Source: CAD feature listing. Evaluate the final solid. Frame: model axes, mm. A direction names the side the tool comes from. Round coordinates to 2 decimals unless told otherwise and drop trailing zeros. Order: outer loops, then holes, each group sorted by start corner. A loop starts at its lowest first (then second) coordinate and runs counter-clockwise, first axis right, second up. Notation, with made-up numbers: (-14.5, 63) - (37.5, 63) arc R11 ccw to (37.5, 81) - close; hole circle Ø11 at (49.25, 25.5). An arc over 180 degrees is marked (long way). Use one line per item in the form item = value. Start each with the question number.
Q1. Ray query, line 1 (X direction, y = 3.5, z = 0); line 2 (X direction, y = 4.75, z = 2.75); line 3 (Z direction, x = -0.25, y = 3.25). Return the intervals inside material, ascending. Write a range as [from, to].
Q2. Cut plane B-B, the plane x = 0. Return the cut outline in (y, z).
Q3. Pin query (flat end, axial travel): pin 1 Ø2 at (x, z) = (3.5, 5.5) entering from +Y; pin 2 Ø1 at (y, z) = (5.5, -5.5) entering from -X; pin 3 Ø6.5 at (x, z) = (0, 0) entering from +Y; pin 4 Ø1 at (x, y) = (5, 4.5) entering from -Z. Return the tip coordinate at first contact, or that it passes through.
Q4. Cut plane D-D, the plane x = -7. Return the cut outline in (y, z), and give its area (3 significant figures).
Q5. Set-up query: faces 5 (the flat face through (5.5, 3, 7)), 6 (the flat face through (6, 0, 0)). Return all of +Z, -Z, +X, -X, +Y, -Y with unobstructed straight access to the full face (end or side cutting, diameter ignored); none if empty.
Q6. Draft query along X for faces 1 (the cylindrical face through (-0.179, 2.958, -5.497)), 2 (the cylindrical face through (-7.02, 0.57, 7.9)), 3 (the cylindrical face through (-6.766, 2.958, -3.49)), 4 (the cylindrical face through (-0.1, 3, -7.5)). Return one class per face: released by +X, released by -X, zero draft, split by the parting line, or undercut.
Q7. Cut plane A-A, the plane z = 0. Return the cut outline in (x, y), and give its area (3 significant figures).
Q8. Cut plane C-C, the plane z = 2. Return the cut outline in (x, y), and give its area (3 significant figures).
Autodesk Inventor part; units mm, degrees
ref_plane "XZ Plane" through (0, 0, 0) normal (0, 1, 0) x (-1, 0, 0)
ref_plane "XY Plane" through (0, 0, 0) normal (0, 0, 1) x (1, 0, 0)
sketch "Sketch1" plane through (0, 0, 0) normal (0, 1, 0) x (-1, 0, 0)
  circle A0 centre (0, 0) radius 5.5
  circle A1 centre (0, 0) radius 7.5
  line L0 (7.5, 0) -> (-7.5, 0)
  line L1 (-7.5, 0) -> (-7.5, 8.5)
  line L2 (-7.5, 8.5) -> (7.5, 8.5)
  line L3 (7.5, 8.5) -> (7.5, 0)
  line L4 (5.5, 0) -> (-5.5, 0)
  line L5 (-5.5, 0) -> (-5.5, 8.5)
  line L6 (-5.5, 8.5) -> (5.5, 8.5)
  line L7 (5.5, 8.5) -> (5.5, 0)
  line L8 (4, 3.7749) -> (4, 6.3443)
  line L9 (-4, 3.7749) -> (-4, 6.3443)
  line L10 (4, 6.3443) -> (5.5, 6.3443)
  line L11 (-4, 6.3443) -> (-5.5, 6.3443)
  line L12 (-10.5, 0) -> (10.5, 0)
  point P0 (-5.5, 8.5)
  dimension "d0" = 11
  dimension "d1" = 2
  dimension "d3" = 1
  dimension "d4" = 1.5
  dimension "d5" = 1.5
extrude "Extrusion1" add sketch "Sketch1" along normal blind 6 contours L0 A1 A0 | L7 A1 L0 | A0 L8 A1 L7 | L5 A1 L9 A0 | L0 A1 L5 | A1 L7 L2 L3 | A1 L10 L7 | L1 L2 L5 A1 | L5 L11 A1
fillet "Fillet1" radius 1.5 2 edges at (-4, 3, 6.3443) (4, 3, 6.3443)
sketch "Sketch4" plane through (-7.5, 0, 0) normal (-1, 0, 0) x (0, 0, 1)
  line L0 (0, 0) -> (8.5, 0)
  line L1 (8.5, 0) -> (8.5, 6)
  line L2 (0, 6) -> (8.5, 6)
  line L3 (0, 0) -> (0, 6)
  line L4 (0, 0) -> (0, 0)
  line L5 (0, 0) -> (0, 6)
  line L6 (0, 6) -> (0, 6)
  line L7 (0, 0) -> (0, 6)
  line L8 (0, 0) -> (0, 6)
  line L9 (0, 6) -> (0, 0)
  line L10 (0, 0) -> (-3, 0)
  line L11 (-3, 0) -> (-3, 6)
  line L12 (-3, 6) -> (0, 6)
  point P0 (0, 0)
  dimension "d22" = 3
extrude "Extrusion3" add sketch "Sketch4" along normal mid plane 2
fillet "Fillet2" radius 2 2 edges at (-8.5, 3, -3) (-6.8739, 3, -3)
mirror "Mirror1" about plane through (0, 0, 0) normal (1, 0, 0) of "Extrusion3", "Fillet2"
fillet "Fillet5" radius 2 4 edges at (7, 6, 8.5) (7, 0, 8.5) (-7, 6, 8.5) (-7, 0, 8.5)
properties part number "Arm_restriction_clip"
Completed:
q1.line_1 = [-8.5, -5.5], [5.5, 8.5]
q1.line_2 = [-8.5, -4.76], [4.76, 8.5]
q1.line_3 = [-7.5, -5.49]
q2.outline = (0, -7.5) - (6, -7.5) - (6, -5.5) - (0, -5.5) - close
q3.pin_1 = 6
q3.pin_2 = -5.59
q3.pin_3 = through
q3.pin_4 = -6
q4.outline = (0, -3.32) - (6, -3.32) - (6, 6.5) arc R2 ccw to (4, 8.5) - (2, 8.5) arc R2 ccw to (0, 6.5) - close
q4.area = 69.2 mm2
q5.face_5 = +Z, +Y, -Y
q5.face_6 = +Z, -Z, +X, -X, -Y
q6.face_1 = undercut
q6.face_2 = zero draft
q6.face_3 = released by -X
q6.face_4 = split by the parting line
q7.outline = (-8.5, 0) - (-5.5, 0) - (-5.5, 6) - (-8.5, 6) - close; (5.5, 0) - (8.5, 0) - (8.5, 6) - (5.5, 6) - close
q7.area = 36.0 mm2
q8.outline = (-8.5, 0) - (-5.12, 0) - (-5.12, 6) - (-8.5, 6) - close; (5.12, 0) - (8.5, 0) - (8.5, 6) - (5.12, 6) - close
q8.area = 40.5 mm2
